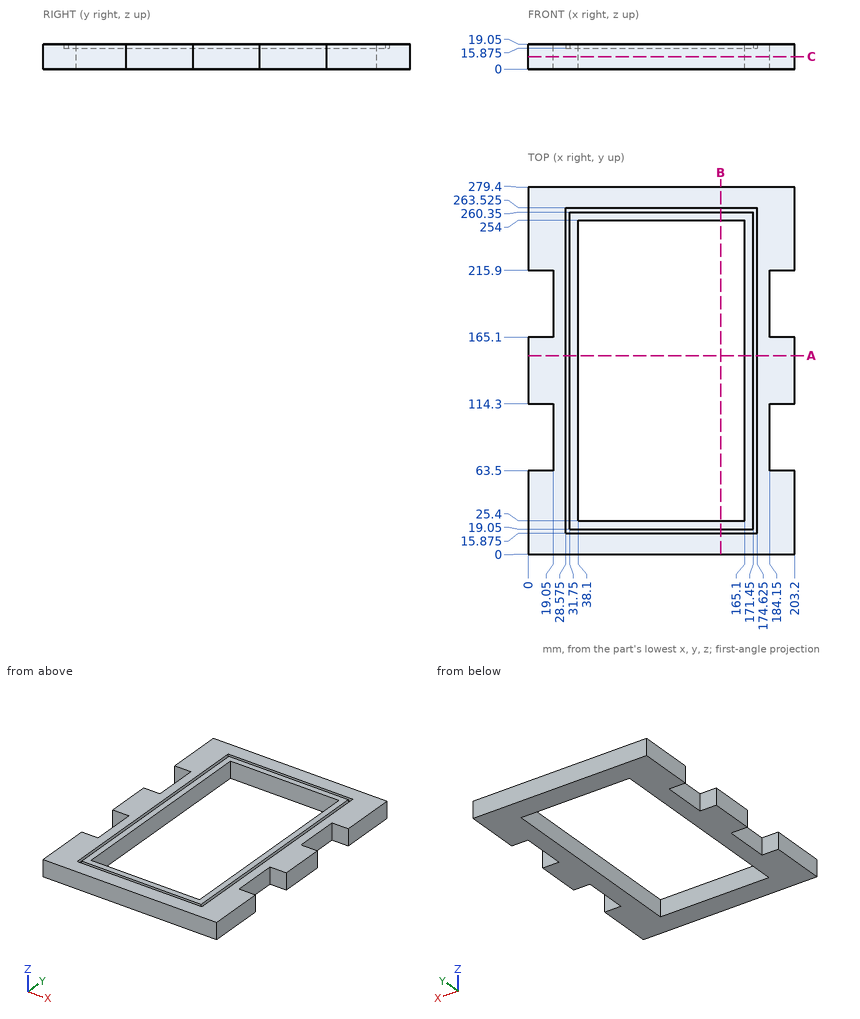
The drawing under review shows one solid part. Ordinate dimensions are in mm from its lowest x, y, z. Coordinates: 2 decimals unless noted, no trailing zeros. Order: outer loops, then holes, each group sorted by start corner. A loop starts at its lowest first (then second) coordinate and runs counter-clockwise, first axis right, second up. Notation, with made-up numbers: (-36.75, 78.25) - (-6.75, 78.25) arc R25 ccw to (-6.75, 112.25) - close; hole circle Ø1 at (14, 6.5). An arc over 180 degrees is marked (long way). Put each result on its own line as item: value.
1) Wall thickness on L1, parallel to X at y = 182, z = 18 (3 decimals); L2, parallel to Y at x = 83, z = 17.25 (3 decimals); L3, parallel to X at y = 246, z = 16.5 (3 decimals): over which ranges is each line inside the solid? List them lowest first. Write a range as from..to.
Response values:
L1: x = 19.05..28.575, 31.75..38.1, 165.1..171.45, 174.625..184.15
L2: y = 0..15.875, 19.05..25.4, 254..260.35, 263.525..279.4
L3: x = 0..28.575, 31.75..38.1, 165.1..171.45, 174.625..203.2
2) Insertion check: P1, Ø10, axis at y = 96, z = 5.5, coming from the +X side; P2, Ø4, axis at x = 29, z = 6, coming from the -Y side; P3, Ø8, axis at y = 179.5, z = 16.5, coming from the -X side. Each pin has a flat end and moves straight along its axis. Give the tip position at first contact, or say it passes through.
Response values:
P1: stops at x = 184.15
P2: stops at y = 0
P3: stops at x = 19.05
3) Take a section at C-C, the plane z = 9.5. Give the boundary of the cut face in (x, y), and give its area (3 significant figures).
Response values:
outline: (0, 0) - (203.2, 0) - (203.2, 63.5) - (184.15, 63.5) - (184.15, 114.3) - (203.2, 114.3) - (203.2, 165.1) - (184.15, 165.1) - (184.15, 215.9) - (203.2, 215.9) - (203.2, 279.4) - (0, 279.4) - (0, 215.9) - (19.05, 215.9) - (19.05, 165.1) - (0, 165.1) - (0, 114.3) - (19.05, 114.3) - (19.05, 63.5) - (0, 63.5) - close; hole (38.1, 25.4) - (165.1, 25.4) - (165.1, 254) - (38.1, 254) - close
area: 23,900 mm²
4) Take a section at B-B, the plane x = 146.5. Give the boundary of the cut face in (y, z) (3 decimals), and give its area (3 significant figures).
Response values:
outline: (0, 0) - (25.4, 0) - (25.4, 19.05) - (19.05, 19.05) - (19.05, 15.875) - (15.875, 15.875) - (15.875, 19.05) - (0, 19.05) - close; (254, 0) - (279.4, 0) - (279.4, 19.05) - (263.525, 19.05) - (263.525, 15.875) - (260.35, 15.875) - (260.35, 19.05) - (254, 19.05) - close
area: 948 mm²
5) Take a section at A-A, the plane y = 151. Give the boundary of the cut face in (x, z) (3 decimals).
Response values:
outline: (0, 0) - (38.1, 0) - (38.1, 19.05) - (31.75, 19.05) - (31.75, 15.875) - (28.575, 15.875) - (28.575, 19.05) - (0, 19.05) - close; (165.1, 0) - (203.2, 0) - (203.2, 19.05) - (174.625, 19.05) - (174.625, 15.875) - (171.45, 15.875) - (171.45, 19.05) - (165.1, 19.05) - close
